from build123d import *

# Parameters (mm, degrees)
SKETCH1_R           = 5.99
BOSS_EXTRUDE1_DEPTH = 7.5
SKETCH2_R           = 2
CUT_EXTRUDE1_DEPTH  = 15
SKETCH3_R           = 2
CUT_EXTRUDE5_DEPTH  = 35


with BuildPart() as part:
    # Sketch1 → Boss-Extrude1 (new, symmetric)
    with BuildSketch(Plane.XY):
        with BuildLine():
            Line((-29, 15), (29, 15))
            ThreePointArc((29, 15), (29.707106781, 14.707106781), (30, 14))
            Line((30, 14), (30, -14))
            ThreePointArc((30, -14), (29.707106781, -14.707106781), (29, -15))
            Line((29, -15), (-29, -15))
            ThreePointArc((-29, -15), (-29.707106781, -14.707106781), (-30, -14))
            Line((-30, -14), (-30, 14))
            ThreePointArc((-30, 14), (-29.707106781, 14.707106781), (-29, 15))
        make_face()
        with Locations((15, 0)):
            Circle(SKETCH1_R, mode=Mode.SUBTRACT)
    extrude(amount=BOSS_EXTRUDE1_DEPTH, both=True)

    # Sketch2 → Cut-Extrude1 (cut)
    with BuildSketch(Plane.ZY.offset(30)):
        with Locations(Location((0, 8, 0), (0, 0, 270))):
            Circle(SKETCH2_R)
        with Locations(Location((0, -8, 0), (0, 0, 270))):
            Circle(SKETCH2_R)
    extrude(amount=-CUT_EXTRUDE1_DEPTH, mode=Mode.SUBTRACT)

    # Sketch3 → Cut-Extrude5 (cut)
    with BuildSketch(Plane(origin=(0, 15, 0), x_dir=(1, 0, 0), z_dir=(0, 1, 0))):
        with Locations(Location((15, 0, 0), (0, 0, 270))):
            Circle(SKETCH3_R)
    extrude(amount=-CUT_EXTRUDE5_DEPTH, mode=Mode.SUBTRACT)


solid = part.part
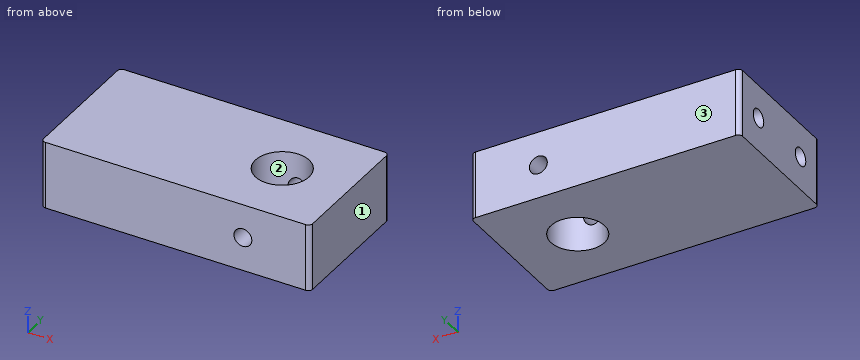
Geometry check sheet. Reference: the model listing, model coordinates, mm. Face numbers are marked on the shaded views. Round coordinates to 2 decimals unless told otherwise and drop trailing zeros. Order: outer loops, then holes, each group sorted by start corner. A loop starts at its lowest first (then second) coordinate and runs counter-clockwise, first axis right, second up. Notation, with made-up numbers: (76.25, 27.25) -> (98.25, 27.25) arc R5 cw to (98.25, 35.25) -> close; hole circle Ø1 at (-34, 79). An arc over 180 degrees is marked (long way). Use one line per item in the form item = value.
1. Cross-section at A-A, the plane y = 0. Enter the section's corners in (x, z), plus the area to 3 significant figures.
Working result:
outline = (-30, -7.5) -> (9.01, -7.5) -> (9.01, 7.5) -> (-30, 7.5) -> close; (20.99, -7.5) -> (30, -7.5) -> (30, 7.5) -> (20.99, 7.5) -> close
area = 720 mm^2
2. Go/stop test with flat-tipped pins: pin 1 (2.5 mm diameter, centred on x = 15, z = 0, fed in from +Y); pin 2 (1.5 mm diameter, centred on y = -9, z = -0.5, fed in from -X). Record where each tip stops, or that it passes through.
Working result:
pin_1 = through
pin_2 = -15
3. Scan lines: line 1 along Z through (x, y) = (15, -11); line 2 along X through (y, z) = (-10.75, 0); line 3 along Z through (x, y) = (16.5, -9). Record each from-to range of solid material in increasing order. Write a range as from..to.
Working result:
line_1 = -7.5..-2, 2..7.5
line_2 = -30..13, 17..30
line_3 = -7.5..-1.32, 1.32..7.5
4. Cross-section at D-D, the plane z = -3.75. Enter the section's corners in (x, y), plus the area to 3 significant figures.
Working result:
outline = (-30, -14) arc R1 ccw to (-29, -15) -> (29, -15) arc R1 ccw to (30, -14) -> (30, 14) arc R1 ccw to (29, 15) -> (-29, 15) arc R1 ccw to (-30, 14) -> close; hole circle Ø11.98 at (15, 0)
area = 1,690 mm^2
5. Cross-section at C-C, the plane x = 15. Enter the section's corners in (y, z).
Working result:
outline = (-15, -7.5) -> (-5.99, -7.5) -> (-5.99, -2) -> (-15, -2) -> close; (-15, 2) -> (-5.99, 2) -> (-5.99, 7.5) -> (-15, 7.5) -> close; (5.99, -7.5) -> (15, -7.5) -> (15, -2) -> (5.99, -2) -> close; (5.99, 2) -> (15, 2) -> (15, 7.5) -> (5.99, 7.5) -> close
6. Cross-section at B-B, the plane z = 0. Enter the section's corners in (x, y).
Working result:
outline = (-30, -14) arc R1 ccw to (-29, -15) -> (13, -15) -> (13, -5.65) arc R5.99 cw to (13, 5.65) -> (13, 15) -> (-29, 15) arc R1 ccw to (-30, 14) -> (-30, 10) -> (-15, 10) -> (-15, 6) -> (-30, 6) -> (-30, -6) -> (-15, -6) -> (-15, -10) -> (-30, -10) -> close; (17, -15) -> (29, -15) arc R1 ccw to (30, -14) -> (30, 14) arc R1 ccw to (29, 15) -> (17, 15) -> (17, 5.65) arc R5.99 cw to (17, -5.65) -> close
7. Mould release check, pull along Y, two halves, no side actions. Record for the marked faces 1, 2 and 3: pulls with the +Y half, pulls with the -Y half, needs draft (parallel to the pull), parting line crosses it, or undercut.
Working result:
face_1 = needs draft
face_2 = undercut
face_3 = pulls with the +Y half
